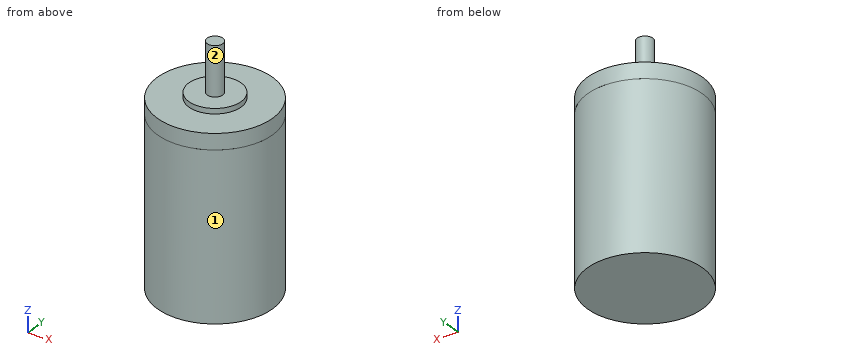
```python
from build123d import *

# Parameters (mm, degrees)
SKETCH1_R      = 11
SKETCH1_R_2    = 5
SKETCH1_R_3    = 1.5
BODY_DEPTH     = 34.5
SKETCH1_3_R    = 5
SKETCH1_3_R_2  = 1.5
COLLAR_DEPTH   = 1
SKETCH1_4_R    = 1.5
SHAFT_DEPTH    = 10.3
CAP_START      = -3
SKETCH2_R      = 11
SKETCH2_R_2    = 10.5
CAP_RING_DEPTH = 0.001


with BuildPart() as part:
    # Sketch1 → Body (new body)
    # profile 1 of 3: a face of its own
    with BuildSketch(Plane.XY):
        Circle(SKETCH1_R)
        Circle(SKETCH1_R_2, mode=Mode.SUBTRACT)
    # profile 2 of 3: a face of its own
    with BuildSketch(Plane.XY):
        Circle(SKETCH1_R_2)
        Circle(SKETCH1_R_3, mode=Mode.SUBTRACT)
    # profile 3 of 3: a face of its own
    with BuildSketch(Plane.XY):
        Circle(SKETCH1_R_3)
    extrude(amount=-BODY_DEPTH)

    # Sketch1_3 → Collar (add)
    # profile 1 of 2: a face of its own
    with BuildSketch(Plane.XY):
        Circle(SKETCH1_3_R)
        Circle(SKETCH1_3_R_2, mode=Mode.SUBTRACT)
    # profile 2 of 2: a face of its own
    with BuildSketch(Plane.XY):
        Circle(SKETCH1_3_R_2)
    extrude(amount=COLLAR_DEPTH)

    # Sketch1_4 → Shaft (add)
    with BuildSketch(Plane.XY):
        with Locations(Location((0, 0, 0), (0, 0, 180))):
            Circle(SKETCH1_4_R)
    extrude(amount=SHAFT_DEPTH)

    # Sketch2 → Cap Ring (cut)
    with BuildSketch(Plane.XY.offset(CAP_START)):
        Circle(SKETCH2_R)
        Circle(SKETCH2_R_2, mode=Mode.SUBTRACT)
    extrude(amount=-CAP_RING_DEPTH, mode=Mode.SUBTRACT)


solid = part.part
```
Model file for the job. Use its own axes, mm. Face numbers are marked on the shaded views. A direction names the side the tool comes from. Coordinates: 2 decimals unless noted, no trailing zeros. Order: outer loops, then holes, each group sorted by start corner. A loop starts at its lowest first (then second) coordinate and runs counter-clockwise, first axis right, second up. Notation, with made-up numbers: M -24.5,74 L 25.5,74 A16 ccw 25.5,98 Z; hole C -1.5,-10 d11. An arc over 180 degrees is marked long. Answer as CSV lines item,"result".
(1) Wall check: line 1 along Z through (x, y) = (7, -5.25); line 2 along Y through (x, z) = (0, -26.5); line 3 along Z through (x, y) = (2, 0.75). Give the ranges that are in metal, low to high.
Geometry says:
line 1,"z = -34.5 to 0"
line 2,"y = -11 to 11"
line 3,"z = -34.5 to 1"
(2) 3-axis set-ups, long thin cutter, end or side, ignore diameter. For the marked faces 1 and 2: which of +Z, -Z, +X, -X, +Y, -Y reach the whole face in a straight line?
Geometry says:
face 1,"+Z, -Z"
face 2,"+Z"
(3) Flat gauge pins, fed straight in: pin 1 (12 mm diameter, centred on y = -3.5, z = 5.5, fed in from -X); pin 2 (3 mm diameter, centred on x = 2.5, y = 2, fed in from +Z); pin 3 (4 mm diameter, centred on x = 2, z = -26.5, fed in from +Y); pin 4 (3 mm diameter, centred on x = 6.5, z = -17, fed in from +Y). Where does each tip first touch, or does it go through?
Geometry says:
pin 1,"stops at x = -10.94"
pin 2,"stops at z = 1"
pin 3,"stops at y = 11"
pin 4,"stops at y = 9.8"
(4) Band-saw the part on C-C, the plane z = 6. List the corners of the cut face in (x, y), then the cut area to 3 significant figures.
Geometry says:
outline,"C 0,0 d3"
area,"7.07 mm2"
